```python
from build123d import *

# Parameters (mm, degrees)
F1_DEPTH = 25.4
F3_DEPTH = 7.1374
F5_DEPTH = 7.1374


with BuildPart() as f1:
    # F0 (on Front) → F1 (new body)
    with BuildSketch(Plane.XZ):
        with BuildLine():
            ThreePointArc((23.749, 9.35351), (-16.807393, 26.132263), (0.040503, -14.395455))
            ThreePointArc((0.040503, -14.395455), (16.807393, -7.425243), (23.749, 9.35351))
        make_face()
        Polygon((47.816977, 47.453566), (-47.433023, 47.453566), (-47.433023, -28.746434), (0.064977, -28.746434), (47.816977, -28.746434), align=None)
        with BuildLine():
            ThreePointArc((23.749, 9.35351), (16.807393, -7.425243), (0.040503, -14.395455))
            ThreePointArc((0.040503, -14.395455), (-16.807393, 26.132263), (23.749, 9.35351))
        make_face(mode=Mode.SUBTRACT)
    extrude(amount=-F1_DEPTH)

    # F2 (on face) → F3 (cut)
    with BuildSketch(Plane.XY.offset(47.453566)):
        with BuildLine():
            ThreePointArc((-31.164323, 12.7), (-34.733023, 16.2687), (-38.301723, 12.7))
            Line((-38.301723, 12.7), (-34.733023, 12.7))
            Line((-34.733023, 12.7), (-31.164323, 12.7))
        make_face()
        with BuildLine():
            Line((-34.733023, 12.7), (-38.301723, 12.7))
            ThreePointArc((-38.301723, 12.7), (-34.733023, 9.1313), (-31.164323, 12.7))
            Line((-31.164323, 12.7), (-34.733023, 12.7))
        make_face()
    extrude(amount=-F3_DEPTH, mode=Mode.SUBTRACT)

    # F4 (on face) → F5 (cut)
    with BuildSketch(Plane.XY.offset(47.453566)):
        with BuildLine():
            ThreePointArc((37.898277, 12.7), (41.466977, 9.1313), (45.035677, 12.7))
            ThreePointArc((45.035677, 12.7), (41.466977, 16.2687), (37.898277, 12.7))
        make_face()
    extrude(amount=-F5_DEPTH, mode=Mode.SUBTRACT)


solid = f1.part
```
Build history of the part. All positions in model axes, mm. A direction names the side the tool comes from. Give positions to 0.01 mm unless a question says otherwise; leave off trailing zeros. Order: outer loops, then holes, each group sorted by start corner. A loop starts at its lowest first (then second) coordinate and runs counter-clockwise, first axis right, second up. Notation, with made-up numbers: M 83.5,62 L 121.5,62 A11 ccw 121.5,80 Z; hole C -4.5,39.5 d1. An arc over 180 degrees is marked long. Return JSON: item names as keys, results as strings.
Q1. Band-saw the part on B-B (x = -2.5). Give the cut face in (y, z).
Answer list:
{"outline": "M 0,-28.75 L 25.4,-28.75 L 25.4,-14.26 L 0,-14.26 Z; M 0,32.97 L 25.4,32.97 L 25.4,47.45 L 0,47.45 Z"}
Q2. Wall check: probe 1 along Z at (x, y) = (0, 18.75); probe 2 along X at (y, z) = (1.5, 29); probe 3 along Z at (x, y) = (5.5, 8). Give the ranges that are in metal, low to high. Write a range as from..to.
Answer list:
{"probe 1": "z = -28.75..-14.4, 33.1..47.45", "probe 2": "x = -47.43..-13.34, 13.34..47.82", "probe 3": "z = -28.75..-13.75, 32.46..47.45"}
Q3. 3-axis set-ups, long thin cutter, end or side, ignore diameter. For faces 1 (the face through (0, 13, -28.746)), 2 (the face through (44.764, 11.333, 43.935)): which of +Z, -Z, +X, -X, +Y, -Y reach the whole face in a straight line?
Answer list:
{"face 1": "-Z, +X, -X, +Y, -Y", "face 2": "+Z"}
Q4. Band-saw the part on D-D (y = 1.5). Give the cut face in (x, z), then the cut area to 3 significant figures.
Answer list:
{"outline": "M -47.43,-28.75 L 47.82,-28.75 L 47.82,47.45 L -47.43,47.45 Z; hole M 0.04,-14.4 A23.75 ccw 23.75,9.35 A23.75 ccw long Z", "area": "5,490 mm^2"}
Q5. Two-plate mould, pull along Y, no slides. Class faces 3 (the face through (47.817, 13, 9)), 4 (the face through (0, 25.4, 35)), 5 (the face through (0, 0, 35)), 6 (the face through (-31.168, 12.543, 43.935)): pulls with the +Y half, pulls with the -Y half, needs draft (parallel to the pull), parting line crosses it, or undercut.
Answer list:
{"face 3": "needs draft", "face 4": "pulls with the +Y half", "face 5": "pulls with the -Y half", "face 6": "undercut"}
Q6. Band-saw the part on A-A (y = 12.7). Give the cut face in (x, z).
Answer list:
{"outline": "M -47.43,-28.75 L 47.82,-28.75 L 47.82,47.45 L 45.04,47.45 L 45.04,40.32 L 37.9,40.32 L 37.9,47.45 L -31.16,47.45 L -31.16,40.32 L -38.3,40.32 L -38.3,47.45 L -47.43,47.45 Z; hole M 0.04,-14.4 A23.75 ccw 23.75,9.35 A23.75 ccw long Z"}
Q7. Flat gauge pin, fed straight in: pin 1 (3.5 mm diameter, centred on x = 42.5, y = 13, fed in from +Z). Where does the tip first touch, or does it go through?
Answer list:
{"pin 1": "stops at z = 40.32"}
Q8. Band-saw the part on C-C (z = 26). Give the cut face in (x, y).
Answer list:
{"outline": "M -47.43,0 L -16.94,0 L -16.94,25.4 L -47.43,25.4 Z; M 16.94,0 L 47.82,0 L 47.82,25.4 L 16.94,25.4 Z"}
